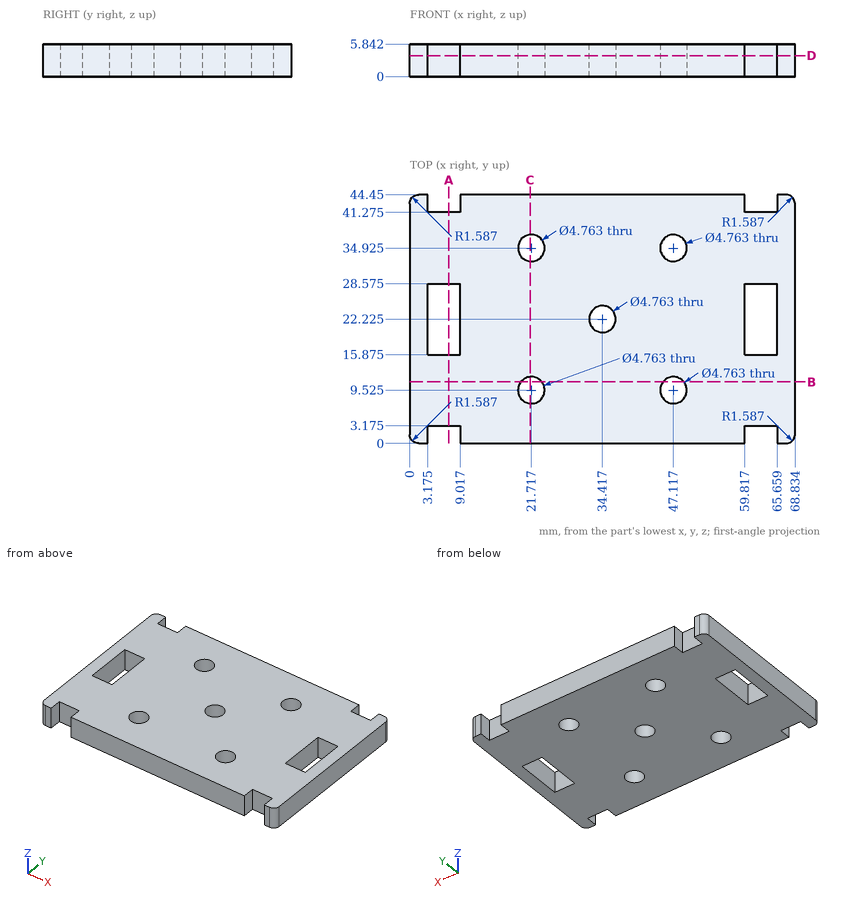
Can you work these out from the drawing? Everything is in mm from the part's minimum corner. Give positions to 0.01 mm unless a question says otherwise; leave off trailing zeros. Order: outer loops, then holes, each group sorted by start corner. A loop starts at its lowest first (then second) coordinate and runs counter-clockwise, first axis right, second up.
1. Suppose I cut it at A-A (x = 7). List the corners of the cut face in (y, z) for me (1 decimal), plus the area to 3 significant figures.
2. Will this pin go through, and if not, where does the flat tip stop? P1, Ø1.8, axis at x = 64, z = 3.5, coming from the -Y side (1 decimal).
3. Suppose I cut it at C-C (x = 21.5). List the corners of the cut face in (y, z) for me.
4. I need wall thicknesses on L1, parallel to X at y = 43, z = 4.45 (1 decimal); L2, parallel to Y at x = 62, z = 0.4 (1 decimal); L3, parallel to X at y = 34.5, z = 2.25 (1 decimal). Which ranges of each line are inside material? Lowest first, please.
5. Suppose I cut it at D-D (z = 3.75). Give the number of separate pieces and of enclosed holes in the cut face, plus the area to 3 significant figures.
6. Suppose I cut it at B-B (y = 11). List the corners of the cut face in (x, z) for me (1 decimal).
Solved:
1. outline: (3.2, 0) - (15.9, 0) - (15.9, 5.8) - (3.2, 5.8) - close; (28.6, 0) - (41.3, 0) - (41.3, 5.8) - (28.6, 5.8) - close
1. area: 148 mm2
2. P1: stops at y = 3.2
3. outline: (0, 0) - (7.15, 0) - (7.15, 5.84) - (0, 5.84) - close; (11.9, 0) - (32.55, 0) - (32.55, 5.84) - (11.9, 5.84) - close; (37.3, 0) - (44.45, 0) - (44.45, 5.84) - (37.3, 5.84) - close
4. L1: x = 0 to 3.2, 9 to 59.8, 65.7 to 68.8
4. L2: y = 3.2 to 15.9, 28.6 to 41.3
4. L3: x = 0 to 19.4, 24.1 to 44.8, 49.5 to 68.8
5. separate pieces: 1
5. enclosed holes: 7
5. area: 2,750 mm2
6. outline: (0, 0) - (19.8, 0) - (19.8, 5.8) - (0, 5.8) - close; (23.6, 0) - (45.2, 0) - (45.2, 5.8) - (23.6, 5.8) - close; (49, 0) - (68.8, 0) - (68.8, 5.8) - (49, 5.8) - close
